```python
from build123d import *

# Parameters (mm, degrees)
SKETCH1_W           = 10
SKETCH1_H           = 6
BOSS_EXTRUDE1_DEPTH = 40
SKETCH7_W           = 10
SKETCH7_H           = 80
BOSS_EXTRUDE3_DEPTH = 6
SKETCH8_W           = 10
SKETCH8_H           = 6
BOSS_EXTRUDE4_DEPTH = 95
SKETCH9_R           = 1.35
CUT_EXTRUDE3_DEPTH  = 80


with BuildPart() as part:
    # Sketch1 → Boss-Extrude1 (new, symmetric)
    with BuildSketch(Plane(origin=(0, 0, 0), x_dir=(1, 0, 0), z_dir=(0, 1, 0))):
        Rectangle(SKETCH1_W, SKETCH1_H)
    extrude(amount=BOSS_EXTRUDE1_DEPTH, both=True)

    # Sketch7 → Boss-Extrude3 (add)
    with BuildSketch(Plane(origin=(0, 40, 0), x_dir=(1, 0, 0), z_dir=(0, 1, 0))):
        with Locations((0, -43)):
            Rectangle(SKETCH7_W, SKETCH7_H)
    extrude(amount=-BOSS_EXTRUDE3_DEPTH)

    # Sketch8 → Boss-Extrude4 (add)
    with BuildSketch(Plane(origin=(0, 40, 0), x_dir=(1, 0, 0), z_dir=(0, 1, 0))):
        with Locations((0, -86)):
            Rectangle(SKETCH8_W, SKETCH8_H)
    extrude(amount=-BOSS_EXTRUDE4_DEPTH)

    # Sketch9 → Cut-Extrude3 (cut)
    with BuildSketch(Plane(origin=(5, 0, 0), x_dir=(0, 0, -1), z_dir=(1, 0, 0))):
        with Locations((-86, -43)):
            Circle(SKETCH9_R)
    extrude(amount=-CUT_EXTRUDE3_DEPTH, mode=Mode.SUBTRACT)


solid = part.part
```
Geometry: final body of the model. Coordinates: model frame, mm. A direction names the side the tool comes from. Coordinates: 2 decimals unless noted, no trailing zeros. Order: outer loops, then holes, each group sorted by start corner. A loop starts at its lowest first (then second) coordinate and runs counter-clockwise, first axis right, second up. Notation, with made-up numbers: (83.25, 71) -> (132.25, 71) arc R12 ccw to (132.25, 94) -> close; hole circle Ø2 at (23.5, 40.5). An arc over 180 degrees is marked (long way). Write item = value, one per line.
(1) Cut plane A-A on y = -32.5. Return loops of the section in (x, z).
Solved:
outline = (-5, -3) -> (5, -3) -> (5, 3) -> (-5, 3) -> close; (-5, 83) -> (5, 83) -> (5, 89) -> (-5, 89) -> close
(2) Access query for faces 1 (the flat face through (0, -10, 83)), 2 (the flat face through (-5, 35, 47)), 3 (the flat face through (0, -40, 0)). Directions: +Z, -Z, +X, -X, +Y, -Y. A direction counts if a zero-diameter tool reaches every point of the face in a straight line with its end or side. Return the directions, or none.
Solved:
face_1 = +X, -X, -Y
face_2 = +Z, -Z, -X, +Y, -Y
face_3 = -Z, +X, -X, -Y
(3) Cut plane B-B on z = 86. Return loops of the section in (x, y).
Solved:
outline = (-5, -55) -> (5, -55) -> (5, -44.35) -> (-5, -44.35) -> close; (-5, -41.65) -> (5, -41.65) -> (5, 40) -> (-5, 40) -> close
(4) Line query: line 1 (Z direction, x = 2.5, y = -28); line 2 (Y direction, x = 1.5, z = 86); line 3 (Y direction, x = -3.25, z = 12.5). Output: solid intervals per line, ascending.
Solved:
line_1 = -3 to 3, 83 to 89
line_2 = -55 to -44.35, -41.65 to 40
line_3 = 34 to 40
(5) Pull-direction query (Z, two-part tool) for faces 4 (the cylindrical face through (0.07, -44.2, 85.38)), 5 (the flat face through (0, 40, 42)), 6 (the flat face through (0, 1, -3)); classes: pulls with the +Z half, pulls with the -Z half, needs draft (parallel to the pull), parting line crosses it, or undercut.
Solved:
face_4 = undercut
face_5 = needs draft
face_6 = pulls with the -Z half
(6) Cut plane D-D on z = 6. Return loops of the section in (x, y).
Solved:
outline = (-5, 34) -> (5, 34) -> (5, 40) -> (-5, 40) -> close
(7) Cut plane C-C on x = -3.5. Return loops of the section in (y, z), plus the area to 3 significant figures.
Solved:
outline = (-55, 83) -> (34, 83) -> (34, 3) -> (-40, 3) -> (-40, -3) -> (40, -3) -> (40, 89) -> (-55, 89) -> close; hole circle Ø2.7 at (-43, 86)
area = 1,520 mm²
(8) Pin query (flat end, axial travel): pin 1 Ø1 at (x, z) = (0, 63) entering from -Y; pin 2 Ø3 at (x, z) = (1, -1.5) entering from -Y; pin 3 Ø2 at (y, z) = (-43, 86) entering from -X. Return the tip coordinate at first contact, or that it passes through.
Solved:
pin_1 = 34
pin_2 = -40
pin_3 = through
